Source: three-view drawing plus pictorial views. Frame: mm from the lowest corner of the part. Coordinates: 2 decimals unless noted, no trailing zeros. Loops run counter-clockwise (first coordinate to the right, second up) from the corner with the lowest first, then second, coordinate; pieces in that order, holes last. Notation, with made-up numbers: M 46.5,87 L 50.5,87 A26 ccw 50.5,110 Z; hole C 52.25,-26 d2. An arc over 180 degrees is marked long. Use a Markdown table: item, result. Add a question column.
1. Section B-B on y = 293.5. Output: boundary loops of the cut face in (x, z), then the cut area to 3 significant figures.
2. Pin query (flat end, axial travel): pin 1 (1 mm diameter, centred on x = 309, y = 263, fed in from -Z); pin 2 (4.5 mm diameter, centred on y = 5.5, z = 13, fed in from +X); pin 3 (3 mm diameter, centred on x = 312, y = 18, fed in from +Z); pin 4 (2 mm diameter, centred on x = 339, z = 8, fed in from -Y). Return the tip coordinate at first contact, or that it passes through.
3. Section C-C on x = 340. Output: boundary loops of the cut face in (y, z).
4. Line query: L1, parallel to Y at x = 18.5, z = 14.25; L2, parallel to X at y = 138.5, z = 6.75; L3, parallel to Y at x = 349, z = 7.5. Output: solid intervals per line, ascending. Write a range as [from, to].
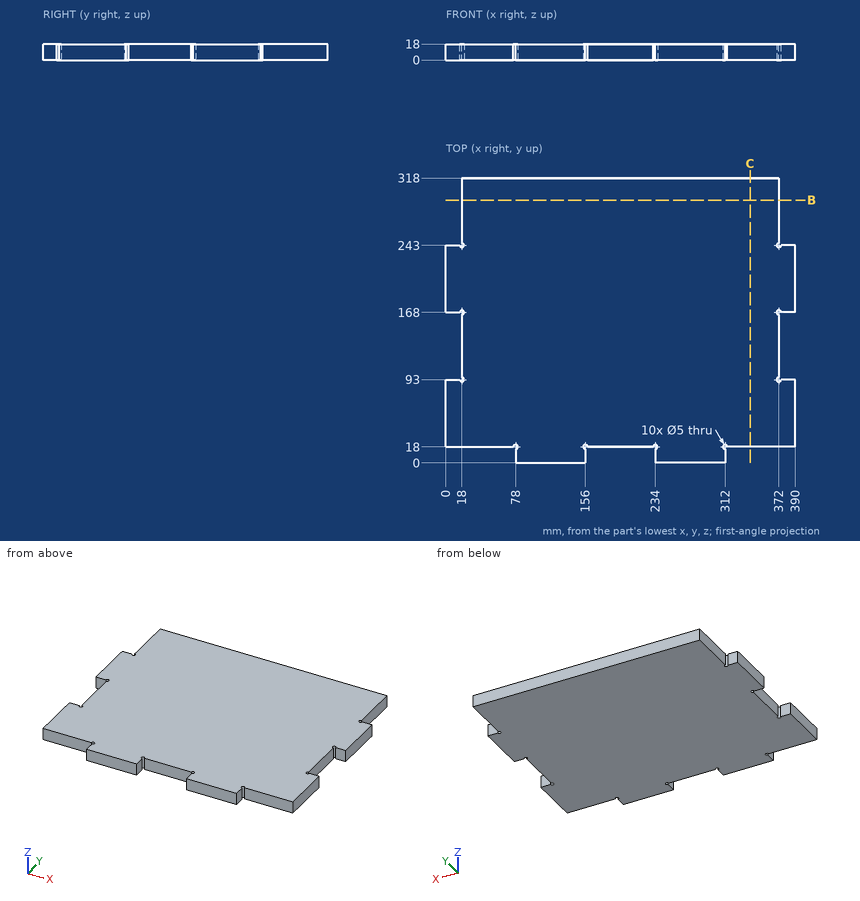
Answers below:
| question | item | result |
|---|---|---|
| 1 | outline | M 18,0 L 372,0 L 372,18 L 18,18 Z |
| 1 | area | 6,370 mm² |
| 2 | pin 1 | stops at z = 0 |
| 2 | pin 2 | stops at x = 312 |
| 2 | pin 3 | passes through |
| 2 | pin 4 | stops at y = 18 |
| 3 | outline | M 18,0 L 318,0 L 318,18 L 18,18 Z |
| 4 | L1 | y = [18, 90.55], [95.45, 165.55], [170.45, 240.55], [245.45, 318] |
| 4 | L2 | x = [18, 372] |
| 4 | L3 | y = [18, 318] |
